from build123d import *

# Parameters (mm, degrees)
SKETCH1_R           = 2
SKETCH1_W           = 4
SKETCH1_H           = 10
BOSS_EXTRUDE1_DEPTH = 4


with BuildPart() as part:
    # Sketch1 → Boss-Extrude1 (new body)
    with BuildSketch(Plane(origin=(0, 0, 0), x_dir=(1, 0, 0), z_dir=(0, 1, 0))):
        Polygon((0, 0), (20, 0), (27.5, 0), (27.5, 4), (42.5, 4), (42.5, 0), (50, 0), (70, 0), (70, 24), (0, 24), align=None)
        with Locations(Location((10, 17, 0), (0, 0, 270))):
            Circle(SKETCH1_R, mode=Mode.SUBTRACT)
        with Locations(Location((60, 17, 0), (0, 0, 90))):
            Circle(SKETCH1_R, mode=Mode.SUBTRACT)
        with Locations((20, 14)):
            Rectangle(SKETCH1_W, SKETCH1_H, mode=Mode.SUBTRACT)
        with Locations((50, 14)):
            Rectangle(SKETCH1_W, SKETCH1_H, mode=Mode.SUBTRACT)
    extrude(amount=BOSS_EXTRUDE1_DEPTH)


solid = part.part
Geometry check sheet. Reference: the model listing, model coordinates, mm. A direction names the side the tool comes from. Round coordinates to 2 decimals unless told otherwise and drop trailing zeros. Write each loop counter-clockwise with the first axis right and the second up, starting at its lowest first coordinate (ties: lowest second). Pieces come first, ordered by that corner, then holes. Notation, with made-up numbers: (81, 79) -> (98, 79) arc R30 cw to (98, 115) -> close; hole circle Ø9 at (-7.5, 51.25). An arc over 180 degrees is marked (long way). One line per item, written item: value. Start each with the question number.
(1) Cross-section at C-C, the plane y = 1.3. Record the cut outline in (x, z), and give its area (3 significant figures).
(2) Go/stop test with flat-tipped pins: pin 1 Ø3 at (x, z) = (34.5, -4.5) entering from -Y; pin 2 Ø2.5 at (x, z) = (10, -17) entering from +Y. Record where each tip stops, or that it passes through.
(3) Access from +Z, -Z, +X, -X, +Y, -Y to the whole of each face (thin tool, end or side, straight path). Record for faces 1 (the flat face through (35, 2, -4)), 2 (the flat face through (70, 2, -12)), 3 (the flat face through (50, 2, -9)).
(4) Cross-section at B-B, the plane z = -3.25. Record the cut outline in (x, y), and give its area (3 significant figures).
(5) Cross-section at A-A, the plane x = 60. Record the cut outline in (y, z), and give its area (3 significant figures).
(6) Scan lines: line 1 (X direction, y = 3, z = -17); line 2 (X direction, y = 2.75, z = -9.75); line 3 (Z direction, x = 60, y = 1.25). Record each from-to range of solid material in increasing order. Write a range as [from, to].
(7) Cross-section at D-D, the plane z = -17. Record the cut outline in (x, y), and give its area (3 significant figures).
(8) Draft check along Z on faces 4 (the flat face through (27.5, 2, -2)), 5 (the flat face through (35, 2, -24)), 6 (the flat face through (48, 2, -14)). Enter one of: +Z half, -Z half, draft (parallel to the pull), parting line (faces both ways), or undercut.
Answer:
1. outline: (0, -24) -> (70, -24) -> (70, 0) -> (42.5, 0) -> (42.5, -4) -> (27.5, -4) -> (27.5, 0) -> (0, 0) -> close; hole circle Ø4 at (10, -17); hole (18, -19) -> (22, -19) -> (22, -9) -> (18, -9) -> close; hole (48, -19) -> (52, -19) -> (52, -9) -> (48, -9) -> close; hole circle Ø4 at (60, -17)
1. area: 1,510 mm²
2. pin 1: y = 0
2. pin 2: through
3. face 1: +Z, +Y, -Y
3. face 2: +Z, -Z, +X, +Y, -Y
3. face 3: +Y, -Y
4. outline: (0, 0) -> (27.5, 0) -> (27.5, 4) -> (0, 4) -> close; (42.5, 0) -> (70, 0) -> (70, 4) -> (42.5, 4) -> close
4. area: 220 mm²
5. outline: (0, -24) -> (4, -24) -> (4, -19) -> (0, -19) -> close; (0, -15) -> (4, -15) -> (4, 0) -> (0, 0) -> close
5. area: 80.0 mm²
6. line 1: [0, 8], [12, 18], [22, 48], [52, 58], [62, 70]
6. line 2: [0, 18], [22, 48], [52, 70]
6. line 3: [-24, -19], [-15, 0]
7. outline: (0, 0) -> (8, 0) -> (8, 4) -> (0, 4) -> close; (12, 0) -> (18, 0) -> (18, 4) -> (12, 4) -> close; (22, 0) -> (48, 0) -> (48, 4) -> (22, 4) -> close; (52, 0) -> (58, 0) -> (58, 4) -> (52, 4) -> close; (62, 0) -> (70, 0) -> (70, 4) -> (62, 4) -> close
7. area: 216 mm²
8. face 4: draft
8. face 5: -Z half
8. face 6: undercut
